The listing builds one solid part. Answer for the finished solid, in the listing's coordinates (mm). A direction names the side the tool comes from. Round coordinates to 2 decimals unless told otherwise and drop trailing zeros. Order: outer loops, then holes, each group sorted by start corner. A loop starts at its lowest first (then second) coordinate and runs counter-clockwise, first axis right, second up. Notation, with made-up numbers: (47, 65.5) - (89, 65.5) arc R33 ccw to (89, 104.5) - close; hole circle Ø4 at (48.5, 38.25). An arc over 180 degrees is marked (long way). One line per item, written item: value. Start each with the question number.
1. Straight lines are drawn through the part: line 1 (Y direction, x = 25.4, z = 94.75) (3 decimals); line 2 (Z direction, x = 13, y = 5.25) (3 decimals); line 3 (Y direction, x = 25, z = 89) (3 decimals). For each, find the intervals that lie inside material, in ascending order.
2. Flat-ended cylindrical pins translate along their axes: P1, Ø5, axis at x = 25.4, y = 0, coming from the +Z side (3 decimals); P2, Ø5, axis at x = -25.4, y = 0, coming from the -Z side (3 decimals); P3, Ø4, axis at y = 6.5, z = 31, coming from the -X side. Find the tip coordinate at first contact, or state that the pin passes through.
3. Section A-A, the plane x = -25.4 is taken. Give the vertices of the cut face in (y, z) (3 decimals).
4. For a pull along X with two mould halves and no side action, classify faces 1 (the flat face through (-25, 0, 85.725)), 2 (the flat face through (1, 0, 98.425)), 3 (the flat face through (50.8, 0, 1)), 4 (the flat face through (27.77, 2.53, -25.49)) as released by +X, released by -X, zero draft, split by the parting line, or undercut.
5. A tool of negligible diameter and unlimited length cuts with its end or side. For faces 5 (the cylindrical face through (-22.37, 0.95, 92.16)), 6 (the flat face through (1, 0, -98.425)), 7 (the flat face through (27.77, 2.53, 25.31)), 8 (the flat face through (-25, 0, -85.725)), 9 (the cylindrical face through (-48.89, -7.714, 1.378)), from which of +Z, -Z, +X, -X, +Y, -Y can it reach the whole face along a straight path? Write none if from no direction.
6. Section B-B, the plane y = 0 is taken. Count the separate pieces of the cut face and the enclosed holes in it, then the cut area to 3 significant figures.
from build123d import *

# Parameters (mm, degrees)
BOSS_EXTRUDE1_DEPTH = 98.425
SKETCH2_R           = 3.175
CUT_EXTRUDE1_DEPTH  = 12.7
SKETCH3_R           = 6.35
CUT_EXTRUDE2_DEPTH  = 66.04


with BuildPart() as part:
    # Sketch1 → Boss-Extrude1 (new body, symmetric)
    with BuildSketch(Plane.XY):
        with BuildLine():
            Line((44.45, 9.525), (50.8, 9.525))
            Line((50.8, 9.525), (50.8, 3.175))
            Line((50.8, 3.175), (50.8, -3.175))
            Line((50.8, -3.175), (50.8, -9.525))
            Line((50.8, -9.525), (44.45, -9.525))
            Line((44.45, -9.525), (-44.45, -9.525))
            ThreePointArc((-44.45, -9.525), (-48.940128061, -7.665128061), (-50.8, -3.175))
            Line((-50.8, -3.175), (-50.8, 3.175))
            ThreePointArc((-50.8, 3.175), (-48.940128061, 7.665128061), (-44.45, 9.525))
            Line((-44.45, 9.525), (44.45, 9.525))
        make_face()
    extrude(amount=BOSS_EXTRUDE1_DEPTH, both=True)

    # Sketch2 → Cut-Extrude1 (cut)
    with BuildSketch(Plane.XY.offset(98.425)):
        with Locations((-25.4, 0)):
            Circle(SKETCH2_R)
        with Locations((25.4, 0)):
            Circle(SKETCH2_R)
    cut_extrude1 = extrude(amount=-CUT_EXTRUDE1_DEPTH, mode=Mode.SUBTRACT)

    # Sketch3 → Cut-Extrude2 (cut)
    with BuildSketch(Plane(origin=(-37.461945986, 21.628664599, 0), x_dir=(0, 0, -1), z_dir=(0.866025404, -0.5, 0))):
        with Locations(Location((-25.4, 15.982254693, 0), (0, 0, 270))):  # turned: the seam where the file's is
            Circle(SKETCH3_R)
        with Locations(Location((25.4, 15.982254693, 0), (0, 0, 270))):  # turned: the seam where the file's is
            Circle(SKETCH3_R)
    extrude(amount=CUT_EXTRUDE2_DEPTH, mode=Mode.SUBTRACT)

    # Mirror1: Cut-Extrude1 across plane
    add(cut_extrude1.mirror(Plane.XY), mode=Mode.SUBTRACT)


solid = part.part
Answer list:
1. line 1: y = -9.525 to -3.175, 3.175 to 9.525
1. line 2: z = -98.425 to -29.395, -21.405 to 21.405, 29.395 to 98.425
1. line 3: y = -9.525 to -3.15, 3.15 to 9.525
2. P1: stops at z = 85.725
2. P2: stops at z = -85.725
2. P3: stops at x = -50.66
3. outline: (-9.525, -98.425) - (-3.175, -98.425) - (-3.175, -85.725) - (3.175, -85.725) - (3.175, -98.425) - (9.525, -98.425) - (9.525, 98.425) - (3.175, 98.425) - (3.175, 85.725) - (-3.175, 85.725) - (-3.175, 98.425) - (-9.525, 98.425) - close
4. face 1: undercut
4. face 2: zero draft
4. face 3: released by +X
4. face 4: undercut
5. face 5: +Z
5. face 6: -Z, +X, -X, +Y, -Y
5. face 7: none
5. face 8: -Z
5. face 9: +Z, -Z, -X, -Y
6. separate pieces: 1
6. enclosed holes: 2
6. area: 19,600 mm²
